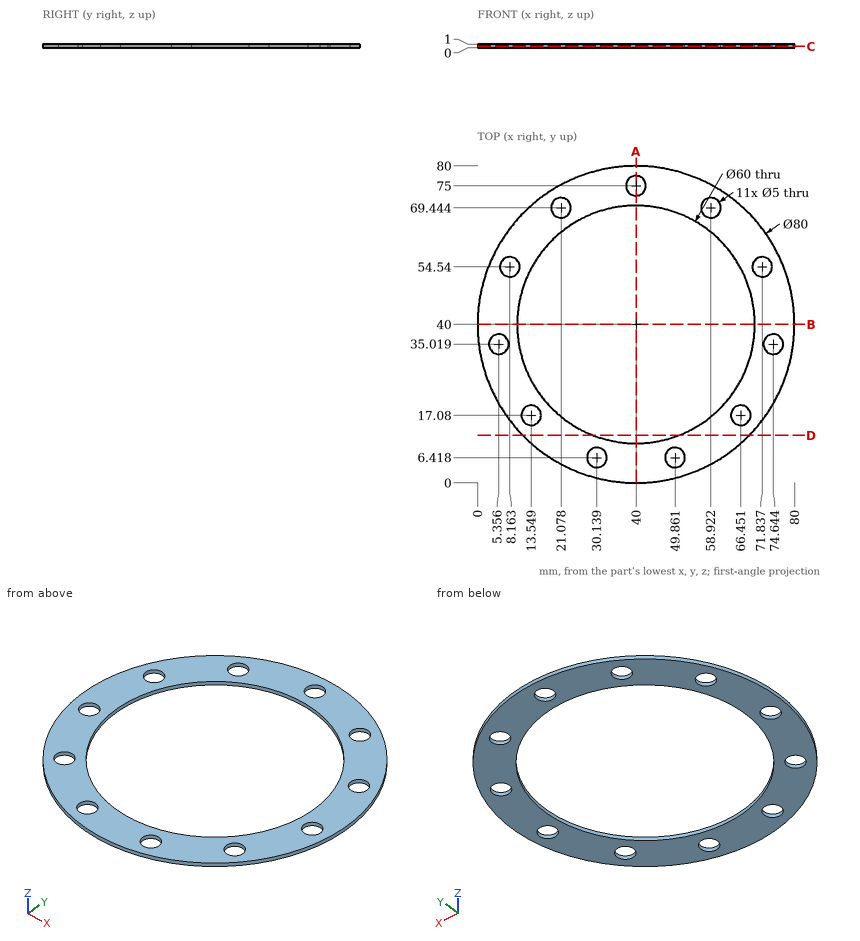
The drawing under review shows one solid part. Ordinate dimensions are in mm from its lowest x, y, z. Coordinates: 2 decimals unless noted, no trailing zeros. Write each loop counter-clockwise with the first axis right and the second up, starting at its lowest first coordinate (ties: lowest second). Pieces come first, ordered by that corner, then holes. Notation, with made-up numbers: M -16,37 L 36,37 A28 cw 36,59 Z; hole C -36,27 d10. An arc over 180 degrees is marked long. Put each result on its own line as item: value.
1) Add section B-B on y = 40. Give the boundary of the cut face in (x, z), then the cut area to 3 significant figures.
Computed:
outline: M 0,0 L 10,0 L 10,1 L 0,1 Z; M 70,0 L 80,0 L 80,1 L 70,1 Z
area: 20.0 mm2
2) Add section A-A on x = 40. Give the boundary of the cut face in (y, z), then the cut area to 3 significant figures.
Computed:
outline: M 0,0 L 10,0 L 10,1 L 0,1 Z; M 70,0 L 72.5,0 L 72.5,1 L 70,1 Z; M 77.5,0 L 80,0 L 80,1 L 77.5,1 Z
area: 15.0 mm2
3) Add section C-C on z = 0.4. State how many separate pieces and enclosed holes the cut face has, then the cut area to 3 significant figures.
Computed:
separate pieces: 1
enclosed holes: 12
area: 1,980 mm2
4) Add section D-D on y = 12. Give the boundary of the cut face in (x, z) (1 decimal).
Computed:
outline: M 11.4,0 L 29.2,0 L 29.2,1 L 11.4,1 Z; M 50.8,0 L 68.6,0 L 68.6,1 L 50.8,1 Z
5) Wall thickness on probe 1 along Y at (x, z) = (50, 0.25) (1 decimal); probe 2 along Y at (x, z) = (49, 0.6) (1 decimal); probe 3 along X at (y, z) = (33, 0.1) (1 decimal): over which ranges is each line inside the solid? List them lowest first. Write a range as [from, to].
Computed:
probe 1: y = [1.3, 3.9], [8.9, 11.7], [68.3, 78.7]
probe 2: y = [1, 4.1], [8.8, 11.4], [68.6, 79]
probe 3: x = [0.6, 3.9], [6.8, 10.8], [69.2, 73.2], [76.1, 79.4]
